from build123d import *

# Parameters (mm, degrees)
F0_W           = 200
F0_H           = 200
F1_DEPTH       = 4
F2_D           = 6.6
F3_D           = 5.5
F3_CSINK_D     = 11.2
F3_CSINK_ANGLE = 90


with BuildPart() as f1:
    # F0 (on Front) → F1 (new body)
    with BuildSketch(Plane.XZ):
        Rectangle(F0_W, F0_H)
    extrude(amount=F1_DEPTH)

    # F2 (through all)
    with Locations(Plane(origin=(0, 0, 0), x_dir=(1, 0, 0), z_dir=(0, 1, 0))):
        with Locations((-45, 0), (45, 0)):
            Hole(F2_D / 2)

    # F3 (through all)
    with Locations(Plane(origin=(0, 0, 0), x_dir=(1, 0, 0), z_dir=(0, 1, 0))):
        with Locations((-90, -90), (90, -90), (-90, 90), (90, 90)):
            CounterSinkHole(F3_D / 2, F3_CSINK_D / 2, counter_sink_angle=F3_CSINK_ANGLE)


solid = f1.part
Verification items for the finished model (mm, model axes). Coordinates: 2 decimals unless noted, no trailing zeros. Order: outer loops, then holes, each group sorted by start corner. A loop starts at its lowest first (then second) coordinate and runs counter-clockwise, first axis right, second up. Notation, with made-up numbers: M 15,20.5 L 35,20.5 A25 cw 35,50.5 Z; hole C 72,40.5 d3. An arc over 180 degrees is marked long. One line per item, written item: value. Start each with the question number.
Item 1: Depth check by flat-ended pin: P1, Ø1, axis at x = -25, z = -33.5, coming from the +Y side. Enter the tip coordinate at first touch or a pass-through.
Item 2: Thickness scan on probe 1 along X at (y, z) = (-3.55, -90); probe 2 along Z at (x, y) = (45, -2.5). Record the ranges inside material, lowest first.
Item 3: Sectioned sample at A-A on z = 0. Record the cut outline in (x, y), then the cut area to 3 significant figures.
Item 4: Mould release check, pull along Z, two halves, no side actions. Record for faces 1 (the flat face through (-1, -4, 1)), 2 (the cylindrical face through (-87.818, -3.433, 91.673)): pulls with the +Z half, pulls with the -Z half, needs draft (parallel to the pull), parting line crosses it, or undercut.
Item 5: Sectioned sample at D-D on z = 90. Record the cut outline in (x, y), then the cut area to 3 significant figures.
Item 6: Sectioned sample at B-B on x = 90. Record the cut outline in (y, z), then the cut area to 3 significant figures.
Item 7: Sectioned sample at C-C on x = 45. Record the cut outline in (y, z), then the cut area to 3 significant figures.
Calculated:
1. P1: y = 0
2. probe 1: -100 to -92.75, -87.25 to 87.25, 92.75 to 100
2. probe 2: -100 to -3.3, 3.3 to 100
3. outline: M -100,-4 L -48.3,-4 L -48.3,0 L -100,0 Z; M -41.7,-4 L 41.7,-4 L 41.7,0 L -41.7,0 Z; M 48.3,-4 L 100,-4 L 100,0 L 48.3,0 Z
3. area: 747 mm^2
4. face 1: needs draft
4. face 2: undercut
5. outline: M -100,-4 L -92.75,-4 L -92.75,-2.85 L -95.6,0 L -100,0 Z; M -87.25,-4 L 87.25,-4 L 87.25,-2.85 L 84.4,0 L -84.4,0 L -87.25,-2.85 Z; M 92.75,-4 L 100,-4 L 100,0 L 95.6,0 L 92.75,-2.85 Z
5. area: 740 mm^2
6. outline: M -4,-100 L 0,-100 L 0,-95.6 L -2.85,-92.75 L -4,-92.75 Z; M -4,-87.25 L -2.85,-87.25 L 0,-84.4 L 0,84.4 L -2.85,87.25 L -4,87.25 Z; M -4,92.75 L -2.85,92.75 L 0,95.6 L 0,100 L -4,100 Z
6. area: 740 mm^2
7. outline: M -4,-100 L 0,-100 L 0,-3.3 L -4,-3.3 Z; M -4,3.3 L 0,3.3 L 0,100 L -4,100 Z
7. area: 774 mm^2
